Can you work these out from the model? Positions are in its coordinate system, mm. A direction names the side the tool comes from. Coordinates: 2 decimals unless noted, no trailing zeros. Loops run counter-clockwise (first coordinate to the right, second up) from the corner with the lowest first, then second, coordinate; pieces in that order, holes last. Notation, with made-up numbers: (55, 42.5) -> (109, 42.5) arc R22 ccw to (109, 51.5) -> close; hole circle Ø3 at (-38, 18.25). An arc over 180 degrees is marked (long way). Use one line per item in the form item = value. Start each with the question number.
(1) Imagine slicing it at A-A (y = 5.25). List the corners of the cut face in (x, z) for me.
(2) I need wall thicknesses on line 1 (X direction, y = 12.5, z = 0); line 2 (Y direction, x = 8.25, z = -1); line 3 (Z direction, x = -5.25, y = 9.5). Which ranges of each line are inside material? Lowest first, please. Write a range as [from, to].
(3) Thinking about a two-plate mould opening in X: for faces 1 (the flat face through (0, 2, 0)), 2 (the flat face through (-10, 1, 0)), 3 (the flat face through (10, 1, 0)), 4 (the flat face through (0, 9, 4.5)), which applies, released by +X, released by -X, zero draft, split by the parting line, or undercut?
(4) On a 3-axis mill with a long thin cutter (end or side, diameter ignored), from which of +Z, -Z, +X, -X, +Y, -Y can I reach the whole of each face in a straight line? I mean faces 5 (the flat face through (6, 9, 0)), 6 (the flat face through (0, 9, -4.5)), 7 (the cylindrical face through (0.9, 8.9, 2.86)). Say none if no direction works.
(5) Imagine slicing it at D-D (x = 0). List the corners of the cut face in (y, z) for me, plus the area to 3 significant figures.
(6) Imagine slicing it at B-B (z = 0). List the corners of the cut face in (x, y) for me, plus the area to 3 significant figures.
(7) I'm going to push flat-ended pins straight in: pin 1 (1.5 mm diameter, centred on x = 4, z = -1, fed in from -Y); pin 2 (7 mm diameter, centred on y = 8, z = -1.5, fed in from -X); pin 3 (2 mm diameter, centred on x = -5.5, z = 7, fed in from +Y); pin 4 (5 mm diameter, centred on y = 10.5, z = -8, fed in from -X). Where does each tip first touch, or does it pass through?
(8) Imagine slicing it at C-C (x = -5.5). List the corners of the cut face in (y, z) for me, plus the area to 3 significant figures.
```python
from build123d import *

# Parameters (mm, degrees)
SKETCH_1_W      = 20
SKETCH_1_H      = 20
EXTRUDE_1_DEPTH = 2
SKETCH_2_W      = 12
SKETCH_2_H      = 9
SKETCH_2_R      = 3
EXTRUDE_2_DEPTH = 14


with BuildPart() as part:
    # 草图1 → 凸台-拉伸1 (new body)
    with BuildSketch(Plane(origin=(0, 0, 0), x_dir=(1, 0, 0), z_dir=(0, 1, 0))):
        Rectangle(SKETCH_1_W, SKETCH_1_H)
    extrude(amount=EXTRUDE_1_DEPTH)

    # 草图2 → 凸台-拉伸2 (add)
    with BuildSketch(Plane(origin=(0, 2, 0), x_dir=(1, 0, 0), z_dir=(0, 1, 0))):
        Rectangle(SKETCH_2_W, SKETCH_2_H)
        with Locations(Location((0, 0, 0), (0, 0, 270))):
            Circle(SKETCH_2_R, mode=Mode.SUBTRACT)
    extrude(amount=EXTRUDE_2_DEPTH)


solid = part.part
```
Worked out:
q1.outline = (-6, -4.5) -> (6, -4.5) -> (6, 4.5) -> (-6, 4.5) -> close; hole circle Ø6 at (0, 0)
q2.line_1 = [-6, -3], [3, 6]
q2.line_2 = [0, 2]
q2.line_3 = [-4.5, 4.5]
q3.face_1 = undercut
q3.face_2 = released by -X
q3.face_3 = released by +X
q3.face_4 = zero draft
q4.face_5 = +Z, -Z, +X, +Y
q4.face_6 = -Z, +X, -X, +Y
q4.face_7 = +Y
q5.outline = (0, -10) -> (2, -10) -> (2, -4.5) -> (16, -4.5) -> (16, -3) -> (2, -3) -> (2, 3) -> (16, 3) -> (16, 4.5) -> (2, 4.5) -> (2, 10) -> (0, 10) -> close
q5.area = 82.0 mm2
q6.outline = (-10, 0) -> (10, 0) -> (10, 2) -> (6, 2) -> (6, 16) -> (3, 16) -> (3, 2) -> (-3, 2) -> (-3, 16) -> (-6, 16) -> (-6, 2) -> (-10, 2) -> close
q6.area = 124 mm2
q7.pin_1 = 0
q7.pin_2 = -6
q7.pin_3 = 2
q7.pin_4 = through
q8.outline = (0, -10) -> (2, -10) -> (2, -4.5) -> (16, -4.5) -> (16, 4.5) -> (2, 4.5) -> (2, 10) -> (0, 10) -> close
q8.area = 166 mm2
